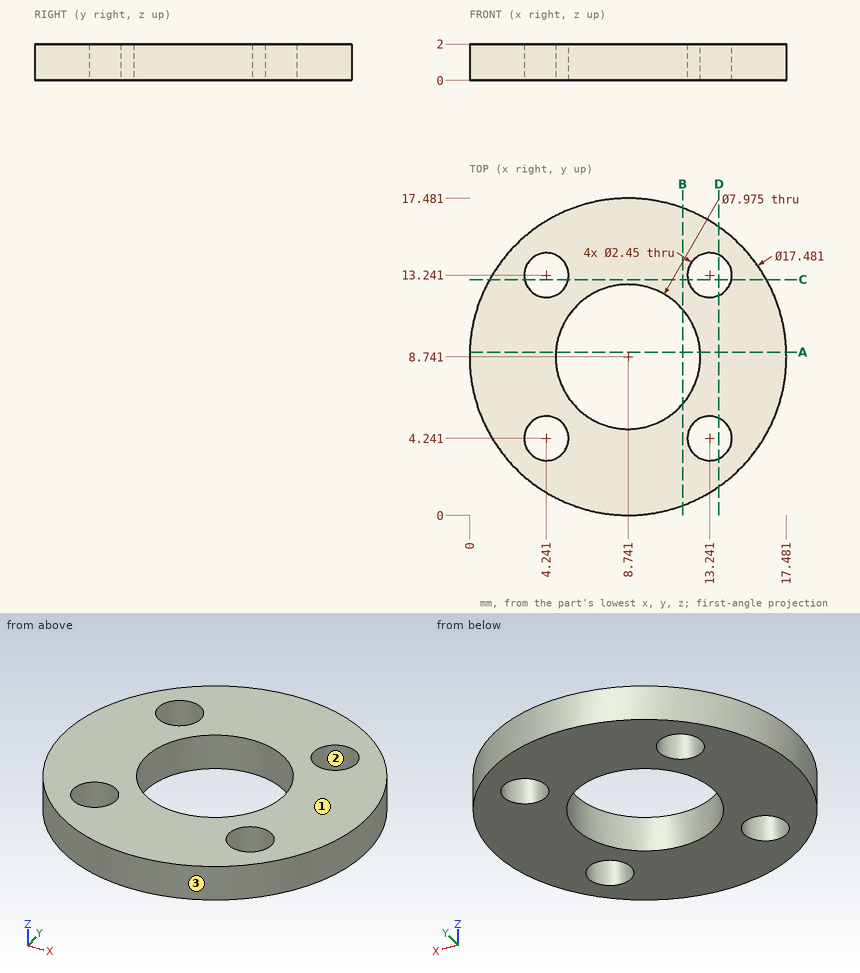
Source: three-view drawing plus pictorial views. Frame: mm from the lowest corner of the part. Round coordinates to 2 decimals unless told otherwise and drop trailing zeros. Write each loop counter-clockwise with the first axis right and the second up, starting at its lowest first coordinate (ties: lowest second). Pieces come first, ordered by that corner, then holes. Notation, with made-up numbers: M 87.25,21.5 L 111.25,21.5 A18 cw 111.25,43.5 Z; hole C -0.75,-28.5 d2. An arc over 180 degrees is marked long. Use CSV: the item, a comma, the result in double quotes. Start each with the question number.
Q1. Cut plane B-B on x = 11.75. Output: boundary loops of the cut face in (y, z) (1 decimal).
Q2. Cut plane D-D on x = 13.75. Output: boundary loops of the cut face in (y, z) (1 decimal).
Q3. Cut plane C-C on y = 13. Output: boundary loops of the cut face in (x, z), plus the area to 3 significant figures.
Q4. Pull-direction query (Y, two-part tool) for the marked faces 1, 2 and 3; classes: +Y half, -Y half, draft (parallel to the pull), parting line (faces both ways), or undercut.
Q5. Cut plane A-A on y = 9. Output: boundary loops of the cut face in (x, z).
Q6. First-contact query: P1, Ø2, axis at x = 4.24, y = 13.24, coming from the -Z side; P2, Ø1, axis at y = 15, z = 1, coming from the +X side (1 decimal); P3, Ø1, axis at y = 10.5, z = 0.5, coming from the +X side. Flat tips, straight axial feed; report the tip coordinate or a pass-through.
Q7. Line query: line 1 (X direction, y = 3.5, z = 0.3) (1 decimal); line 2 (X direction, y = 13.75, z = 1.4) (1 decimal); line 3 (Y direction, x = 13.5, z = 0.85) (1 decimal). Output: solid intervals per line, ascending. Write a range as from..to.
Results found:
1,outline,"M 0.5,0 L 6.1,0 L 6.1,2 L 0.5,2 Z; M 11.4,0 L 16.9,0 L 16.9,2 L 11.4,2 Z"
2,outline,"M 1.6,0 L 3.1,0 L 3.1,2 L 1.6,2 Z; M 5.4,0 L 12.1,0 L 12.1,2 L 5.4,2 Z; M 14.4,0 L 15.9,0 L 15.9,2 L 14.4,2 Z"
3,outline,"M 1.11,0 L 3.04,0 L 3.04,2 L 1.11,2 Z; M 5.44,0 L 12.04,0 L 12.04,2 L 5.44,2 Z; M 14.44,0 L 16.37,0 L 16.37,2 L 14.44,2 Z"
3,area,"20.9 mm^2"
4,face 1,"draft"
4,face 2,"undercut"
4,face 3,"parting line"
5,outline,"M 0,0 L 4.76,0 L 4.76,2 L 0,2 Z; M 12.72,0 L 17.48,0 L 17.48,2 L 12.72,2 Z"
6,P1,"through"
6,P2,"x = 15.3"
6,P3,"x = 17.39"
7,line 1,"1.7..3.3, 5.2..12.3, 14.2..15.7"
7,line 2,"1.6..3.1, 5.4..12.1, 14.4..15.9"
7,line 3,"1.4..3, 5.4..12, 14.4..16.1"
